Model file for the job. Use its own axes, mm. A direction names the side the tool comes from. Round coordinates to 2 decimals unless told otherwise and drop trailing zeros. Loops run counter-clockwise (first coordinate to the right, second up) from the corner with the lowest first, then second, coordinate; pieces in that order, holes last. Notation, with made-up numbers: M 65,7 L 121,7 A17 cw 121,13 Z; hole C -20.75,18 d11. An arc over 180 degrees is marked long. Answer in a Markdown table with one row per item.
from build123d import *

# Parameters (mm, degrees)
SKETCH1_W           = 82.55
SKETCH1_H           = 93.98
BOSS_EXTRUDE1_DEPTH = 1.4732
SKETCH2_W           = 8.636
SKETCH2_H           = 7.62
BOSS_EXTRUDE2_DEPTH = 4.191
SKETCH3_R           = 4.7625
BOSS_EXTRUDE3_DEPTH = 3.6068


with BuildPart() as part:
    # Sketch1 → Boss-Extrude1 (new body)
    with BuildSketch(Plane(origin=(0, 0, 0), x_dir=(1, 0, 0), z_dir=(0, 1, 0))):
        Rectangle(SKETCH1_W, SKETCH1_H)
    extrude(amount=BOSS_EXTRUDE1_DEPTH)

    # Sketch2 → Boss-Extrude2 (add)
    with BuildSketch(Plane(origin=(0, 0, 0), x_dir=(1, 0, 0), z_dir=(0, 1, 0))):
        with Locations((39.497, -31.75)):
            Rectangle(SKETCH2_W, SKETCH2_H)
    extrude(amount=BOSS_EXTRUDE2_DEPTH)

    # Sketch3 → Boss-Extrude3 (add)
    with BuildSketch(Plane.XZ):
        with Locations(Location((-31.75, 38.1, 0), (0, 0, 270))):
            Circle(SKETCH3_R)
        with Locations(Location((31.75, 38.1, 0), (0, 0, 270))):
            Circle(SKETCH3_R)
        with Locations(Location((-31.75, -38.1, 0), (0, 0, 270))):
            Circle(SKETCH3_R)
        with Locations(Location((31.75, -38.1, 0), (0, 0, 270))):
            Circle(SKETCH3_R)
    extrude(amount=BOSS_EXTRUDE3_DEPTH)


solid = part.part
1. Wall check: probe 1 along Y at (x, z) = (31.5, 16); probe 2 along X at (y, z) = (1, -21.5) (3 decimals); probe 3 along Z at (x, y) = (-32.5, -2). Give the ranges that are in metal, low to high.
Verdict:
| item | result |
|---|---|
| probe 1 | y = 0 to 1.47 |
| probe 2 | x = -41.275 to 41.275 |
| probe 3 | z = -42.8 to -33.4, 33.4 to 42.8 |
2. Saw through at C-C (x = -31.75). Write the cut outline in (y, z), and give its area (3 significant figures).
Verdict:
| item | result |
|---|---|
| outline | M -3.61,-42.86 L 0,-42.86 L 0,-46.99 L 1.47,-46.99 L 1.47,46.99 L 0,46.99 L 0,42.86 L -3.61,42.86 L -3.61,33.34 L 0,33.34 L 0,-33.34 L -3.61,-33.34 Z |
| area | 207 mm² |
3. Saw through at B-B (z = 38.1). Write the cut outline in (x, y) (1 decimal).
Verdict:
| item | result |
|---|---|
| outline | M -41.3,0 L -36.5,0 L -36.5,-3.6 L -27,-3.6 L -27,0 L 27,0 L 27,-3.6 L 36.5,-3.6 L 36.5,0 L 41.3,0 L 41.3,1.5 L -41.3,1.5 Z |
4. Saw through at A-A (y = -1.75). State how many separate pieces and enclosed holes the cut face has, and give its area (3 significant figures).
Verdict:
| item | result |
|---|---|
| separate pieces | 4 |
| enclosed holes | 0 |
| area | 285 mm² |
5. Saw through at D-D (z = -22). Write the cut outline in (x, y) (3 decimals), and give its area (3 significant figures).
Verdict:
| item | result |
|---|---|
| outline | M -41.275,0 L 41.275,0 L 41.275,1.473 L -41.275,1.473 Z |
| area | 122 mm² |
6. Mould opens along X. For faces 4 (the cylindrical face through (31.959, -1.778, 42.858)), 5 (the flat face through (32, -3.607, 38)), 6 (the flat face through (43.815, 2, 32)) say: +X half, -X half, draft (parallel to the pull), parting line (faces both ways), or undercut.
Verdict:
| item | result |
|---|---|
| face 4 | undercut |
| face 5 | draft |
| face 6 | +X half |
7. Pin check, flat tips, straight feed: pin 1 (5 mm diameter, centred on x = 12, z = -32, fed in from -Y); pin 2 (2 mm diameter, centred on x = 39, y = 3, fed in from -Z); pin 3 (2 mm diameter, centred on x = -6, z = -31.5, fed in from +Y). Stop position of each tip, or through.
Verdict:
| item | result |
|---|---|
| pin 1 | stops at y = 0 |
| pin 2 | stops at z = 27.94 |
| pin 3 | stops at y = 1.47 |
8. Tool access for faces 1 (the cylindrical face through (-31.541, -1.778, 42.858)), 2 (the flat face through (32, -3.607, -38)), 3 (the flat face through (35.179, 3, 32)): list every direction of +Z, -Z, +X, -X, +Y, -Y with a clear straight run to the whole face (end or side of a thin tool).
Verdict:
| item | result |
|---|---|
| face 1 | -Y |
| face 2 | +Z, -Z, +X, -X, -Y |
| face 3 | +Z, -Z, -X, +Y |
